Geometry check sheet. Reference: the model listing, model coordinates, mm. Coordinates: 2 decimals unless noted, no trailing zeros. Loops run counter-clockwise (first coordinate to the right, second up) from the corner with the lowest first, then second, coordinate; pieces in that order, holes last. Notation, with made-up numbers: M 53.5,85 L 82.5,85 A12 cw 82.5,99 Z; hole C 76.5,20 d7. An arc over 180 degrees is marked long. One line per question, with ' | ' between items. Start each with the question number.
from build123d import *

# Parameters (mm, degrees)
F0_R     = 2
F1_DEPTH = 0.25


with BuildPart() as f1:
    # F0 (on Top) → F1 (new body, symmetric)
    with BuildSketch(Plane.XY):
        with BuildLine():
            ThreePointArc((-6, -3), (-5.2565835097, -1.5811388301), (-5, 0))
            ThreePointArc((-5, 0), (-5.2565835097, 1.5811388301), (-6, 3))
            ThreePointArc((-6, 3), (-15, 0), (-6, -3))
        make_face()
        with Locations((-10, 0)):
            Circle(F0_R, mode=Mode.SUBTRACT)
        with BuildLine():
            ThreePointArc((15, 0), (11.5811388301, 4.7434164903), (6, 3))
            ThreePointArc((6, 3), (5, 0), (6, -3))
            ThreePointArc((6, -3), (11.5811388301, -4.7434164903), (15, 0))
        make_face()
        with Locations((10, 0)):
            Circle(F0_R, mode=Mode.SUBTRACT)
        with BuildLine():
            ThreePointArc((-6, 3), (-5.2565835097, 1.5811388301), (-5, 0))
            ThreePointArc((-5, 0), (-5.2565835097, -1.5811388301), (-6, -3))
            Line((-6, -3), (6, -3))
            ThreePointArc((6, -3), (5, 0), (6, 3))
            Line((6, 3), (-6, 3))
        make_face()
    extrude(amount=F1_DEPTH, both=True)


solid = f1.part
1. Sectioned sample at B-B (y = -1.25). Record the cut outline in (x, z).
2. Sectioned sample at A-A (x = 10). Record the cut outline in (y, z), and give its area (3 significant figures).
3. Thickness scan on line 1 (Y direction, x = -10, z = 0.2); line 2 (X direction, y = 0.25, z = -0.1); line 3 (Y direction, x = -2, z = -0.05). Record the ranges inside material, lowest first.
4. Sectioned sample at C-C (z = 0.1). Record the cut outline in (x, y), and give its area (3 significant figures).
5. Depth check by flat-ended pin: pin 1 Ø3 at (x, y) = (10, 0) entering from -Z. Enter the tip coordinate at first touch or a pass-through.
6. Sectioned sample at D-D (y = 4.25). Record the cut outline in (x, z), and give its area (3 significant figures).
7. Draft check along X on faces 1 (the cylindrical face through (-15, 0, 0)), 2 (the flat face through (0, 0, 0.25)). Enter one of: +X half, -X half, draft (parallel to the pull), parting line (faces both ways), or undercut.
Result:
1) outline: M -14.84,-0.25 L -11.56,-0.25 L -11.56,0.25 L -14.84,0.25 Z; M -8.44,-0.25 L 8.44,-0.25 L 8.44,0.25 L -8.44,0.25 Z; M 11.56,-0.25 L 14.84,-0.25 L 14.84,0.25 L 11.56,0.25 Z
2) outline: M -5,-0.25 L -2,-0.25 L -2,0.25 L -5,0.25 Z; M 2,-0.25 L 5,-0.25 L 5,0.25 L 2,0.25 Z | area: 3.00 mm2
3) line 1: y = -5 to -2, 2 to 5 | line 2: x = -14.99 to -11.98, -8.02 to 8.02, 11.98 to 14.99 | line 3: y = -3 to 3
4) outline: M -6,-3 L 6,-3 A5 ccw long 6,3 L -6,3 A5 ccw long Z; hole C -10,0 d4; hole C 10,0 d4 | area: 196 mm2
5) pin 1: passes through
6) outline: M -12.63,-0.25 L -7.37,-0.25 L -7.37,0.25 L -12.63,0.25 Z; M 7.37,-0.25 L 12.63,-0.25 L 12.63,0.25 L 7.37,0.25 Z | area: 5.27 mm2
7) face 1: undercut | face 2: draft
